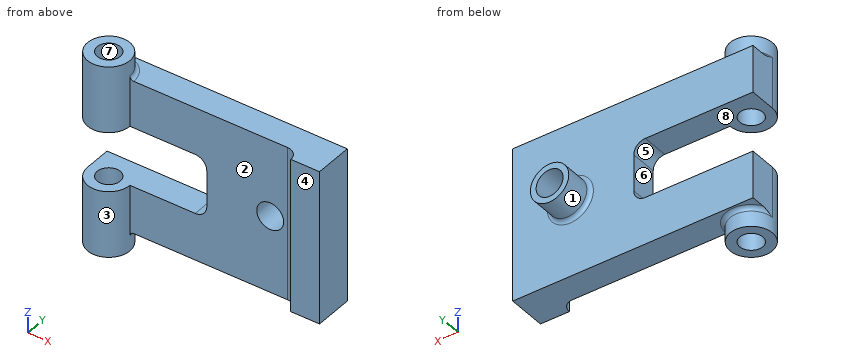
from build123d import *

# Parameters (mm, degrees)
SKETCH1_R           = 6
BOSS_EXTRUDE1_DEPTH = 40
BOSS_EXTRUDE2_DEPTH = 50
SKETCH2_W           = 62
SKETCH2_H           = 31
CUT_EXTRUDE1_DEPTH  = 137.930639376
SKETCH3_R           = 7
CUT_EXTRUDE2_DEPTH  = 137.930639376
BOSS_EXTRUDE3_START = 15
SKETCH3_3_R         = 10
SKETCH3_3_R_2       = 7
BOSS_EXTRUDE3_DEPTH = 15
FILLET1_R           = 6
FILLET2_R           = 2


with BuildPart() as part:
    # Sketch1 → Boss-Extrude1 (new, symmetric)
    with BuildSketch(Plane.XY):
        with BuildLine():
            Line((22, 0), (104, 0))
            ThreePointArc((104, 0), (108.242640687, -1.757359313), (110, -6))
            Line((110, -6), (125, -6))
            Line((125, -6), (125, 14))
            Line((125, 14), (0, 14))
            Line((0, 14), (0, 0))
            ThreePointArc((0, 0), (11, -11), (22, 0))
        make_face()
        with Locations((11, 0)):
            Circle(SKETCH1_R, mode=Mode.SUBTRACT)
    extrude(amount=BOSS_EXTRUDE1_DEPTH, both=True)

    # Sketch1<3> → Boss-Extrude2 (add, symmetric)
    with BuildSketch(Plane.XY):
        with BuildLine():
            ThreePointArc((22, 0), (11, 11), (0, 0))
            Line((0, 0), (5, 0))
            ThreePointArc((5, 0), (11, 6), (17, 0))
            Line((17, 0), (22, 0))
        make_face()
        with BuildLine():
            Line((5, 0), (0, 0))
            ThreePointArc((0, 0), (11, -11), (22, 0))
            Line((22, 0), (17, 0))
            ThreePointArc((17, 0), (11, -6), (5, 0))
        make_face()
    extrude(amount=BOSS_EXTRUDE2_DEPTH, both=True)

    # Sketch2 → Cut-Extrude1 (cut, through all)
    with BuildSketch(Plane(origin=(0, 14, 0), x_dir=(1, 0, 0), z_dir=(0, 1, 0))):
        with Locations((31, 0)):
            Rectangle(SKETCH2_W, SKETCH2_H)
    extrude(amount=-CUT_EXTRUDE1_DEPTH, mode=Mode.SUBTRACT)

    # Sketch3 → Cut-Extrude2 (cut, through all)
    with BuildSketch(Plane(origin=(0, 14, 0), x_dir=(1, 0, 0), z_dir=(0, 1, 0))):
        with Locations(Location((95, 0, 0), (0, 0, 270))):
            Circle(SKETCH3_R)
    extrude(amount=-CUT_EXTRUDE2_DEPTH, mode=Mode.SUBTRACT)

    # Sketch3<3> → Boss-Extrude3 (add)
    with BuildSketch(Plane(origin=(0, 14, 0), x_dir=(1, 0, 0), z_dir=(0, 1, 0)).offset(BOSS_EXTRUDE3_START)):
        with Locations(Location((95, 0, 0), (0, 0, 270))):
            Circle(SKETCH3_3_R)
        with Locations(Location((95, 0, 0), (0, 0, 270))):
            Circle(SKETCH3_3_R_2, mode=Mode.SUBTRACT)
    extrude(amount=-BOSS_EXTRUDE3_DEPTH)

    # Fillet1
    fillet1_edges = [part.edges().sort_by_distance(p)[0] for p in [
        (62, 7, 15.5),
        (62, 7, -15.5),
    ]]
    fillet(fillet1_edges, radius=FILLET1_R)

    # Fillet2
    # the kernel refuses this fillet: 2 mm, written as the material it adds along each edge
    with BuildSketch(Plane(origin=(11, 0, -40), x_dir=(1, 0, 0), z_dir=(0, -1, 0))) as fillet2_piece_1_section:
        with BuildLine():
            CenterArc((11 + FILLET2_R, -FILLET2_R), FILLET2_R, 90, 90)
            Line((11 + FILLET2_R, 0), (11, 0))
            Line((11, 0), (11, -FILLET2_R))
        make_face()
    fillet2_piece_1 = revolve(axis=Axis((11, 0, -40), (0, 0, 1)), revolution_arc=180, mode=Mode.PRIVATE)
    fillet2_piece_1 = split(fillet2_piece_1, bisect_by=Plane(origin=(0, 11.564222142, -40.564222142), z_dir=(1, 0, 0)), keep=Keep.TOP, mode=Mode.PRIVATE)
    add(fillet2_piece_1)
    with BuildSketch(Plane(origin=(11, 0, 40), x_dir=(1, 0, 0), z_dir=(0, -1, 0))) as fillet2_piece_2_section:
        with BuildLine():
            CenterArc((11 + FILLET2_R, FILLET2_R), FILLET2_R, 180, 90)
            Line((11, FILLET2_R), (11, 0))
            Line((11, 0), (11 + FILLET2_R, 0))
        make_face()
    fillet2_piece_2 = revolve(axis=Axis((11, 0, 40), (0, 0, 1)), revolution_arc=180, mode=Mode.PRIVATE)
    fillet2_piece_2 = split(fillet2_piece_2, bisect_by=Plane(origin=(0, 11.564222139, 40.564222139), z_dir=(1, 0, 0)), keep=Keep.TOP, mode=Mode.PRIVATE)
    add(fillet2_piece_2)
    with BuildSketch(Plane(origin=(95, 14, 0), x_dir=(0, 0, 1), z_dir=(-1, 0, 0))) as fillet2_piece_3:
        with BuildLine():
            CenterArc((10 + FILLET2_R, FILLET2_R), FILLET2_R, 180, 90)
            Line((10, FILLET2_R), (10, 0))
            Line((10, 0), (10 + FILLET2_R, 0))
        make_face()
    revolve(axis=Axis((95, 14, 0), (0, 1, 0)))


solid = part.part
Read the model definition and answer for the solid it produces. Units are mm, in the model's axes. Face numbers are marked on the shaded views. A direction names the side the tool comes from. Coordinates: 2 decimals unless noted, no trailing zeros. Loops run counter-clockwise (first coordinate to the right, second up) from the corner with the lowest first, then second, coordinate; pieces in that order, holes last. Notation, with made-up numbers: (53, -12.75) -> (101, -12.75) arc R31 ccw to (101, 15.25) -> close; hole circle Ø3 at (70, 45). An arc over 180 degrees is marked (long way). Write item = value, one per line. Start each with the question number.
1) The part is cut by section B-B, the plane z = 0. Determine the outline of the cut face in (x, y).
2) The part is cut by section D-D, the plane z = 38. Determine the outline of the cut face in (x, y).
3) Find the intervals of material crossed by L1, parallel to X at y = 8, z = 0; L2, parallel to Y at x = 11, z = -32; L3, parallel to Z at x = 9, y = -9, in increasing order. Write a range as from..to.
4) The part is cut by section A-A, the plane x = 31. Determine the outline of the cut face in (y, z), plus the area to 3 significant figures.
5) The part is cut by section C-C, the plane x = 11. Determine the outline of the cut face in (y, z).
6) The mould has two halves that part along X. Classify the marked faces 6, 7 and 8: pulls with the +X half, pulls with the -X half, needs draft (parallel to the pull), parting line crosses it, or undercut.
7) Given P1, Ø2, axis at x = 88, z = 39.5, coming from the +Y side; P2, Ø20, axis at x = 41.5, y = 6.5, coming from the -Z side; P3, Ø12, axis at y = 19.5, z = 0.5, coming from the -X side, each flat-ended and moving along its own axis, determine where each tip first touches the part or whether it passes through.
8) For the marked faces 1, 2, 3, 4 and 5, determine the directions among +Z, -Z, +X, -X, +Y, -Y from which every point of the face is accessible in a straight line to the end or side of a thin tool.
Result:
q1.outline = (62, 0) -> (88, 0) -> (88, 29) -> (85, 29) -> (85, 16) arc R2 cw to (83, 14) -> (62, 14) -> close; (102, 0) -> (104, 0) arc R6 cw to (110, -6) -> (125, -6) -> (125, 14) -> (107, 14) arc R2 cw to (105, 16) -> (105, 29) -> (102, 29) -> close
q2.outline = (0, 0) arc R11 ccw to (22, 0) -> (104, 0) arc R6 cw to (110, -6) -> (125, -6) -> (125, 14) -> (0, 14) -> close; hole circle Ø12 at (11, 0)
q3.L1 = 62..88, 102..125
q3.L2 = -11..-6, 6..14
q3.L3 = -50..-15.5, 15.5..50
q4.outline = (0, -40) -> (14, -40) -> (14, -15.5) -> (0, -15.5) -> close; (0, 15.5) -> (14, 15.5) -> (14, 40) -> (0, 40) -> close
q4.area = 686 mm²
q5.outline = (-11, -50) -> (-6, -50) -> (-6, -15.5) -> (-11, -15.5) -> close; (-11, 15.5) -> (-6, 15.5) -> (-6, 50) -> (-11, 50) -> close; (6, -50) -> (11, -50) -> (11, -42) arc R2 cw to (13, -40) -> (14, -40) -> (14, -15.5) -> (6, -15.5) -> close; (6, 15.5) -> (14, 15.5) -> (14, 40) -> (13, 40) arc R2 cw to (11, 42) -> (11, 50) -> (6, 50) -> close
q6.face_6 = pulls with the -X half
q6.face_7 = undercut
q6.face_8 = needs draft
q7.P1 = 14
q7.P2 = -40
q7.P3 = 62
q8.face_1 = +Y
q8.face_2 = +Z, -Z, -Y
q8.face_3 = -Z
q8.face_4 = +Z, -Z, +X, -Y
q8.face_5 = -X, +Y, -Y
